Read the model definition and answer for the solid it produces. Units are mm, in the model's axes. Coordinates: 2 decimals unless noted, no trailing zeros. Write each loop counter-clockwise with the first axis right and the second up, starting at its lowest first coordinate (ties: lowest second). Pieces come first, ordered by that corner, then holes.
1) Each of these flat-tipped pins is pushed along its axis until it touches: pin 1 Ø1.5 at (y, z) = (-95.5, 0) entering from +X; pin 2 Ø2.5 at (x, z) = (97.5, -1) entering from +Y. Where does it stop, or does it pass through?
2) The part is cut by section C-C (z = 1.75). Determine the outline of the cut face in (x, y).
3) The part is cut by section A-A (x = 111). Determine the outline of the cut face in (y, z).
4) The part is cut by section B-B (x = 88). Determine the outline of the cut face in (y, z).
5) Find the intervals of material crossed by line 1 (Y direction, x = 109, z = 1.55); line 2 (Y direction, x = 101, z = -1); line 3 (X direction, y = -141.5, z = 0.75), in increasing order.
6) The part is cut by section D-D (y = -136.5). Determine the outline of the cut face in (x, z), then the cut area to 3 significant figures.
from build123d import *

# Parameters (mm, degrees)
BOSS_EXTRUDE1_DEPTH = 2.5


with BuildPart() as part:
    # Sketch2 → Boss-Extrude1 (new, symmetric)
    with BuildSketch(Plane.XY):
        Polygon((113.746163942, -98.757408203), (108.496163942, -98.757408203), (108.496163942, -78.257408203), (113.746163942, -78.257408203), (113.746163942, -73.507408203), (103.996163942, -73.507408203), (103.996163942, -78.757408203), (93.496163942, -78.757408203), (93.496163942, -73.507408203), (83.746163942, -73.507408203), (83.746163942, -93.507408203), (88.746163942, -93.507408203), (88.746163942, -134.007377288), (83.746163942, -134.007377288), (83.746163942, -154.007377288), (93.496163942, -154.007377288), (93.496163942, -148.757377288), (103.996163942, -148.757377288), (103.996163942, -154.007377288), (113.746163942, -154.007377288), (113.746163942, -149.257377288), (108.496163942, -149.257377288), (108.496163942, -128.757377288), (113.746163942, -128.757377288), align=None)
    extrude(amount=BOSS_EXTRUDE1_DEPTH, both=True)


solid = part.part
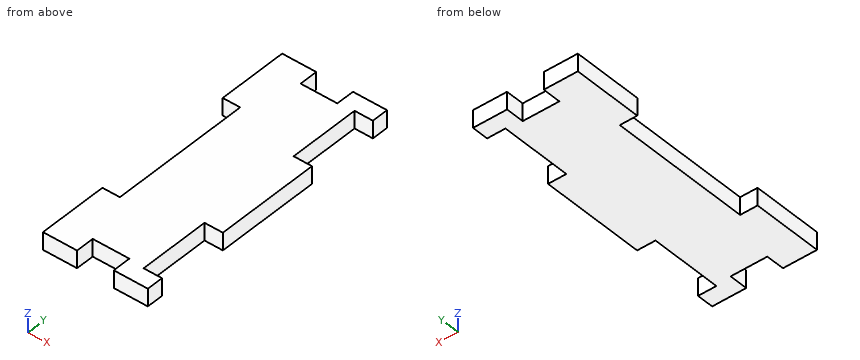
Reported:
1. pin 1: stops at x = 108.5
1. pin 2: stops at y = -78.76
2. outline: (83.75, -154.01) - (93.5, -154.01) - (93.5, -148.76) - (104, -148.76) - (104, -154.01) - (113.75, -154.01) - (113.75, -149.26) - (108.5, -149.26) - (108.5, -128.76) - (113.75, -128.76) - (113.75, -98.76) - (108.5, -98.76) - (108.5, -78.26) - (113.75, -78.26) - (113.75, -73.51) - (104, -73.51) - (104, -78.76) - (93.5, -78.76) - (93.5, -73.51) - (83.75, -73.51) - (83.75, -93.51) - (88.75, -93.51) - (88.75, -134.01) - (83.75, -134.01) - close
3. outline: (-154.01, -2.5) - (-149.26, -2.5) - (-149.26, 2.5) - (-154.01, 2.5) - close; (-128.76, -2.5) - (-98.76, -2.5) - (-98.76, 2.5) - (-128.76, 2.5) - close; (-78.26, -2.5) - (-73.51, -2.5) - (-73.51, 2.5) - (-78.26, 2.5) - close
4. outline: (-154.01, -2.5) - (-134.01, -2.5) - (-134.01, 2.5) - (-154.01, 2.5) - close; (-93.51, -2.5) - (-73.51, -2.5) - (-73.51, 2.5) - (-93.51, 2.5) - close
5. line 1: y = -154.01 to -149.26, -128.76 to -98.76, -78.26 to -73.51
5. line 2: y = -148.76 to -78.76
5. line 3: x = 83.75 to 108.5
6. outline: (83.75, -2.5) - (108.5, -2.5) - (108.5, 2.5) - (83.75, 2.5) - close
6. area: 124 mm2
